Could you check a few things on this drawing? It's one solid part, dimensions in mm from its lowest x, y, z. A direction names the side the tool comes from. Give positions to 0.01 mm unless a question says otherwise; leave off trailing zeros. Write each loop counter-clockwise with the first axis right and the second up, starting at its lowest first coordinate (ties: lowest second). Pieces come first, ordered by that corner, then holes.
1. On a 3-axis mill with a long thin cutter (end or side, diameter ignored), from which of +Z, -Z, +X, -X, +Y, -Y can I reach the whole of each face in a straight line? I mean the marked faces 1, 2 and 3. Say none if no direction works.
2. Suppose I cut it at A-A (z = 0.5). Please give me the cut outline in (x, y), and give its area (3 significant figures).
3. Suppose I cut it at C-C (x = 15). Please give me the cut outline in (y, z), and give its area (3 significant figures).
4. I'm going to push flat-ended pins straight in: pin 1 (1.5 mm diameter, centred on x = 28, z = 2, fed in from -Y); pin 2 (3.5 mm diameter, centred on x = 14, z = 4, fed in from +Y); pin 3 (2 mm diameter, centred on y = 2.5, z = 6, fed in from +X). Where does each tip first touch, or does it pass through?
5. Suppose I cut it at B-B (y = 1.75). Please give me the cut outline in (x, z).
6. If I drill on probe 1 along X at (y, z) = (13.5, 5.5); probe 2 along Y at (x, z) = (4, 6), over which ranges is the centre line in solid material (lowest first)?
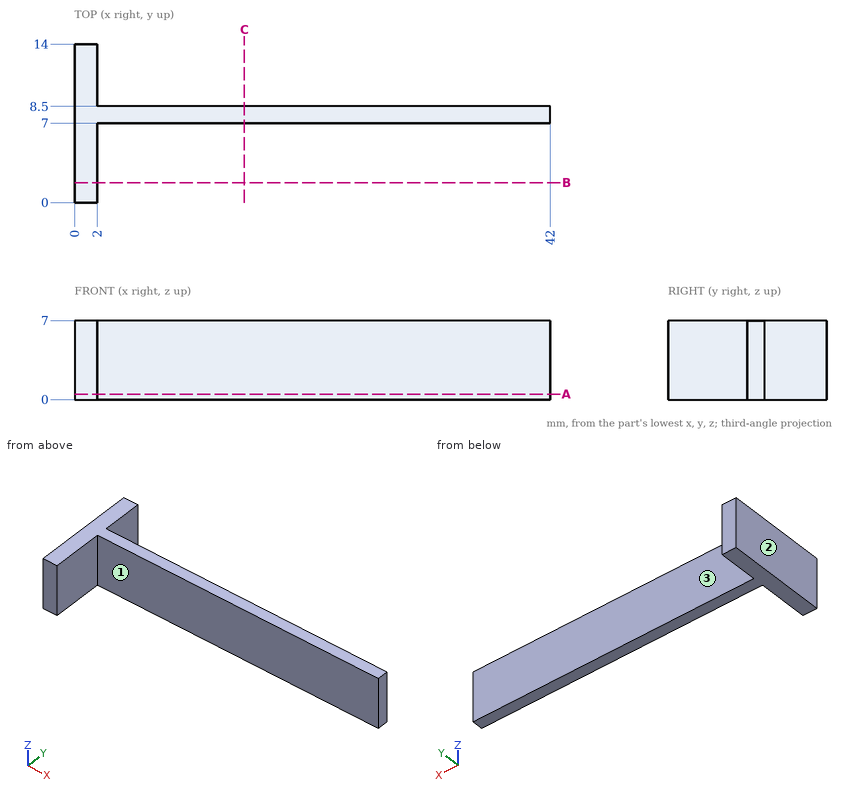
Checks:
1. face 1: +Z, -Z, +X, -Y
1. face 2: +Z, -Z, -X, +Y, -Y
1. face 3: +Z, -Z, +X, +Y
2. outline: (0, 0) - (2, 0) - (2, 7) - (42, 7) - (42, 8.5) - (2, 8.5) - (2, 14) - (0, 14) - close
2. area: 88.0 mm2
3. outline: (7, 0) - (8.5, 0) - (8.5, 7) - (7, 7) - close
3. area: 10.5 mm2
4. pin 1: stops at y = 7
4. pin 2: stops at y = 8.5
4. pin 3: stops at x = 2
5. outline: (0, 0) - (2, 0) - (2, 7) - (0, 7) - close
6. probe 1: x = 0 to 2
6. probe 2: y = 7 to 8.5
